from build123d import *

# Parameters (mm, degrees)
F2_R     = 15.24
F3_DEPTH = 25.4
F4_R     = 17.78
F4_R_2   = 17.272
F5_DEPTH = 25.4


with BuildPart() as f1:
    # F0 (on Front) → F1 (revolve)
    with BuildSketch(Plane.XZ):
        with BuildLine():
            Line((0, 0), (17.78, 0))
            Line((17.78, 0), (17.78, 11.070003))
            ThreePointArc((17.78, 11.070003), (17.126763, 29.27488), (15.170413, 47.38612))
            Line((15.170413, 47.38612), (0, 152.4))
            Line((0, 152.4), (0, 0))
        make_face()
    revolve(axis=Axis((0, 0, 88.9), (0, 0, 1)))

    # F2 (on face) → F3 (cut)
    with BuildSketch(Plane(origin=(0, 0, 0), x_dir=(1, 0, 0), z_dir=(0, 0, -1))):
        Circle(F2_R)
    extrude(amount=-F3_DEPTH, mode=Mode.SUBTRACT)

    # F4 (on face) → F5 (cut)
    with BuildSketch(Plane(origin=(0, 0, 25.4), x_dir=(1, 0, 0), z_dir=(0, 0, -1))):
        Circle(F4_R)
        Circle(F4_R_2, mode=Mode.SUBTRACT)
    extrude(amount=F5_DEPTH, mode=Mode.SUBTRACT)


solid = f1.part
Could you check a few things on this model? Use its own coordinates, in mm. A direction names the side the tool comes from. Give positions to 0.01 mm unless a question says otherwise; leave off trailing zeros. Order: outer loops, then holes, each group sorted by start corner. A loop starts at its lowest first (then second) coordinate and runs counter-clockwise, first axis right, second up. Notation, with made-up numbers: M 83,21.5 L 127,21.5 A36 cw 127,59.5 Z; hole C 36.25,34.25 d11. An arc over 180 degrees is marked long. One line per question, with ' | ' between items.
1. I want a section at A-A (z = 114). List the corners of the cut face in (x, y) for me, and give its area (3 significant figures).
Results:
outline: C 0,0 d11.09 | area: 96.7 mm²
2. If I drill on line 1 (Y direction, x = 0, z = 5.5); line 2 (Y direction, x = 8, z = 24.5), over which ranges is the centre line in solid material (lowest first)?
Results:
line 1: -17.27 to -15.24, 15.24 to 17.27 | line 2: -15.31 to -12.97, 12.97 to 15.31
3. I'm going to push flat-ended pins straight in: pin 1 (1 mm diameter, centred on x = 8, y = -9, fed in from -Z); pin 2 (1 mm diameter, centred on x = 5.5, z = 75, fed in from -Y); pin 3 (8 mm diameter, centred on x = -9.5, z = 95.5, fed in from +Y). Where does each tip first touch, or does it pass through?
Results:
pin 1: z = 25.4 | pin 2: y = -10.01 | pin 3: y = 6.19
4. For faces 1 (the face through (-3.3, 14.88, 12.52)), 2 (the face through (-1.62, -7.3, 100.63)), which set-ups out of +Z, -Z, +X, -X, +Y, -Y let a thin tool reach every point of the face, with its end or its side?
Results:
face 1: -Z | face 2: +Z
5. We'd pull the mould along Y, two halves only. Please class faces 3 (the face through (-9, -13, 0)), 4 (the face through (0, 0, 25.4)), 5 (the face through (-2.248, -17.125, 12.878)): +Y half, -Y half, draft (parallel to the pull), parting line (faces both ways), or undercut.
Results:
face 3: draft | face 4: undercut | face 5: parting line
6. I want a section at B-B (z = 75.5). List the corners of the cut face in (x, y) for me, and give its area (3 significant figures).
Results:
outline: C 0,0 d22.22 | area: 388 mm²
